from build123d import *

# Parameters (mm, degrees)
REVOLVE1_ANGLE                 = 177.5
BOSS_EXTRUDE1_REACH            = 72.435
BOSS_EXTRUDE1_END_MAJOR_RADIUS = 31.55
BOSS_EXTRUDE1_END_MINOR_RADIUS = 2.45
BOSS_EXTRUDE2_DEPTH            = 1.25
BOSS_EXTRUDE3_REACH            = 68.663
BOSS_EXTRUDE3_END_RADIUS       = 31.55
SKETCH7_R                      = 0.5
CUT_EXTRUDE1_DEPTH             = 49.523762708
BOSS_EXTRUDE4_START            = -2.45
BOSS_EXTRUDE4_DEPTH            = 4.9
BOSS_EXTRUDE5_DEPTH            = 4.9
SKETCH11_R                     = 1.05
CUT_EXTRUDE2_DEPTH             = 49.543542798
CHAMFER1_SIZE                  = 0.1
CUT_REVOLVE4_ANGLE             = 5


# Read off the part's stored shape, not the designer's step: Boss-Extrude4
with BuildPart() as part:
    # Sketch1 → Revolve1 (revolve)
    with BuildSketch(Plane(origin=(0, 0, 0), x_dir=(0, 0, -1), z_dir=(1, 0, 0))):
        with BuildLine():
            Line((-1.9, 31.55), (-2.45, 31.55))
            ThreePointArc((-2.45, 31.55), (0, 34), (2.45, 31.55))
            Line((2.45, 31.55), (1.9, 31.55))
            Line((1.9, 31.55), (1.732550899, 32.3))
            ThreePointArc((1.732550899, 32.3), (1.713964889, 32.375442776), (1.692095441, 32.45))
            ThreePointArc((1.692095441, 32.45), (0, 33.306290622), (-1.692095441, 32.45))
            ThreePointArc((-1.692095441, 32.45), (-1.713964889, 32.375442776), (-1.732550899, 32.3))
            Line((-1.732550899, 32.3), (-1.9, 31.55))
        make_face()
    revolve(axis=Axis((0, 0, -25.465534681), (0, 0, 1)), revolution_arc=REVOLVE1_ANGLE)



with BuildPart() as body_2:
    # Boss-Extrude1: up to this torus (the profile starts outside it)
    boss_extrude1_end = Plane(origin=(0, 0, 0), z_dir=(0, 0, -1)) * Torus(BOSS_EXTRUDE1_END_MAJOR_RADIUS, BOSS_EXTRUDE1_END_MINOR_RADIUS, mode=Mode.PRIVATE)
    # Sketch4 → Boss-Extrude1 (new, up to the surface)
    with BuildSketch(Plane(origin=(-11.970705016, 32.889241728, 0), x_dir=(-0.9396926207859083, -0.34202014332566943, 0), z_dir=(0.34202014332566943, -0.9396926207859083, 0)), mode=Mode.PRIVATE) as boss_extrude1_sk1:
        Polygon((3.25, 1.75), (-3.25, 1.5), (-3.25, -1.5), (3.25, -1.75), align=None)
    boss_extrude1_tool1 = extrude(boss_extrude1_sk1.sketch, amount=BOSS_EXTRUDE1_REACH, mode=Mode.PRIVATE) - boss_extrude1_end
    add(boss_extrude1_tool1.solids().sort_by_distance((-12.049013, 32.86074, 0))[0])


with BuildPart() as part_1:
    add(part.part)

    add(body_2.part)  # Boss-Extrude2 merges body 2
    # Sketch5 → Boss-Extrude2 (add, symmetric)
    with BuildSketch(Plane.XY):
        with BuildLine():
            Line((-14.896879867, 32.888378954), (-14.554859724, 31.948686333))
            Line((-14.554859724, 31.948686333), (-9.386550309, 33.829797122))
            Line((-9.386550309, 33.829797122), (-9.557560381, 34.299643432))
            Line((-9.557560381, 34.299643432), (-11.718054934, 33.513287723))
            ThreePointArc((-11.718054934, 33.513287723), (-12.14691319, 33.378696125), (-12.586125644, 33.28316224))
            Line((-12.586125644, 33.28316224), (-14.896879867, 32.888378954))
        make_face()
    extrude(amount=BOSS_EXTRUDE2_DEPTH, both=True)

    # Boss-Extrude3: up to this cylinder (the profile starts outside it)
    boss_extrude3_end = Plane(origin=(0, 0, 0), z_dir=(0, 0, -1)) * Cylinder(BOSS_EXTRUDE3_END_RADIUS, 201.426, mode=Mode.PRIVATE)
    # Sketch6 → Boss-Extrude3 (add, up to the surface)
    with BuildSketch(Plane(origin=(-17.5, 30.310889132, 0), x_dir=(0.866025403784438, 0.5000000000000012, 0), z_dir=(-0.5000000000000012, 0.866025403784438, 0)), mode=Mode.PRIVATE) as boss_extrude3_sk1:
        with BuildLine():
            Line((-0.75, -2.25), (0.75, -2.25))
            ThreePointArc((0.75, -2.25), (1.457106781, -1.957106781), (1.75, -1.25))
            Line((1.75, -1.25), (1.75, 1.25))
            ThreePointArc((1.75, 1.25), (1.457106781, 1.957106781), (0.75, 2.25))
            Line((0.75, 2.25), (-0.75, 2.25))
            ThreePointArc((-0.75, 2.25), (-1.457106781, 1.957106781), (-1.75, 1.25))
            Line((-1.75, 1.25), (-1.75, -1.25))
            ThreePointArc((-1.75, -1.25), (-1.457106781, -1.957106781), (-0.75, -2.25))
        make_face()
    boss_extrude3_tool1 = extrude(boss_extrude3_sk1.sketch, amount=-BOSS_EXTRUDE3_REACH, mode=Mode.PRIVATE) - boss_extrude3_end
    add(boss_extrude3_tool1.solids().sort_by_distance((-17.5, 30.310889, 0))[0])

    # Sketch7 → Cut-Extrude1 (cut, through all)
    with BuildSketch(Plane.XY.offset(2.25)):
        with Locations((-17, 29.444863729)):
            Circle(SKETCH7_R)
    extrude(amount=-CUT_EXTRUDE1_DEPTH, mode=Mode.SUBTRACT)

    # Boss-Extrude4 outline → Boss-Extrude4 (add)
    with BuildSketch(Plane.XY.offset(BOSS_EXTRUDE4_START)):
        with BuildLine():
            Line((-29.900129226, -17.819785976), (-27.005409062, -16.312890038))
            ThreePointArc((-27.005409062, -16.312890038), (-27.985191787, -14.568168747), (-28.852403515, -12.764846705))
            Line((-28.852403515, -12.764846705), (-31.747123679, -14.271742644))
            Line((-31.747123679, -14.271742644), (-29.900129226, -17.819785976))
        make_face()
    extrude(amount=BOSS_EXTRUDE4_DEPTH)

    # Sketch10 → Boss-Extrude5 (add)
    with BuildSketch(Plane.XY.offset(2.45)):
        with BuildLine():
            Line((-31.747123679, -14.271742644), (-29.900129226, -17.819785976))
            ThreePointArc((-29.900129226, -17.819785976), (-32.597648119, -16.969261536), (-31.747123679, -14.271742644))
        make_face()
    extrude(amount=-BOSS_EXTRUDE5_DEPTH)

    # Sketch11 → Cut-Extrude2 (cut, through all)
    with BuildSketch(Plane.XY.offset(2.45)):
        with Locations((-30.823626453, -16.04576431)):
            Circle(SKETCH11_R)
    extrude(amount=-CUT_EXTRUDE2_DEPTH, mode=Mode.SUBTRACT)

    # Chamfer1
    chamfer1_edges = [part_1.edges().sort_by_distance(p)[0] for p in [
        (-31.873626453, -16.04576431, -2.45),
        (-31.873626453, -16.04576431, 2.45),
    ]]
    chamfer(chamfer1_edges, length=CHAMFER1_SIZE)

    # Sketch12 → Cut-Revolve2 (revolve, cut)
    with BuildSketch(Plane(origin=(0, 0, 0), x_dir=(0, 0, -1), z_dir=(1, 0, 0))):
        with BuildLine():
            Line((-1.9, 31.55), (1.9, 31.55))
            Line((1.9, 31.55), (1.732550899, 32.3))
            ThreePointArc((1.732550899, 32.3), (1.713964889, 32.375442776), (1.692095441, 32.45))
            ThreePointArc((1.692095441, 32.45), (0, 33.306290622), (-1.692095441, 32.45))
            ThreePointArc((-1.692095441, 32.45), (-1.713964889, 32.375442776), (-1.732550899, 32.3))
            Line((-1.732550899, 32.3), (-1.9, 31.55))
        make_face()
    revolve(axis=Axis((0, 0, -14.066037571), (0, 0, 1)), mode=Mode.SUBTRACT)

    # Sketch13 → Cut-Revolve4 (revolve, cut)
    with BuildSketch(Plane(origin=(0, 0, 0), x_dir=(0, 0, -1), z_dir=(0.999048221581858, -0.043619387365329415, 0))):
        with BuildLine():
            Line((0, -33.306290622), (0, -34))
            ThreePointArc((0, -34), (1.732411614, -33.282411614), (2.45, -31.55))
            Line((2.45, -31.55), (1.9, -31.55))
            Line((1.9, -31.55), (1.732550899, -32.3))
            ThreePointArc((1.732550899, -32.3), (1.713964889, -32.375442776), (1.692095441, -32.45))
            ThreePointArc((1.692095441, -32.45), (0.948211555, -33.080028823), (0, -33.306290622))
        make_face()
    revolve(axis=Axis((0, 0, -14.693028928), (0, 0, -1)), revolution_arc=CUT_REVOLVE4_ANGLE, mode=Mode.SUBTRACT)


solid = part_1.part
Read the model definition and answer for the solid it produces. Units are mm, in the model's axes. A direction names the side the tool comes from. Round coordinates to 2 decimals unless told otherwise and drop trailing zeros. Write each loop counter-clockwise with the first axis right and the second up, starting at its lowest first coordinate (ties: lowest second). Pieces come first, ordered by that corner, then holes. Notation, with made-up numbers: M 81,-1.5 L 91,-1.5 A13 ccw 91,11.5 Z; hole C -26,87.5 d3. An arc over 180 degrees is marked long. Use a Markdown table: item, result.
1) Flat-ended cylindrical pins translate along their axes: pin 1 (2 mm diameter, centred on x = -29, z = -0.5, fed in from -Y); pin 2 (1.9 mm diameter, centred on x = -11.5, y = 33, fed in from -Z); pin 3 (3 mm diameter, centred on x = -17.5, y = 28.5, fed in from +Z). Find the tip coordinate at first contact, or state that the pin passes through.
Answers follow:
| item | result |
|---|---|
| pin 1 | stops at y = -19.23 |
| pin 2 | stops at z = -1.64 |
| pin 3 | stops at z = 2.42 |
2) The part is cut by section A-A (y = 0). Write down the section's boundary in (x, z).
Answers follow:
| item | result |
|---|---|
| outline | M -32.45,-1.69 A2.1 cw -32.45,1.69 A1.78 cw -32.3,1.73 L -31.55,1.9 L -31.55,2.45 A2.45 ccw -31.55,-2.45 L -31.55,-1.9 L -32.3,-1.73 A1.78 cw Z |
3) Straight lines are drawn through the part: line 1 along Y through (x, z) = (-17, 0.45); line 2 along Y through (x, z) = (-14.5, -0.3); line 3 along Y through (x, z) = (-29, 1.05). For each, find the intervals that lie inside material, in ascending order. Write a range as [from, to].
Answers follow:
| item | result |
|---|---|
| line 1 | y = [-29.4, -28.58], [28.58, 28.94], [29.94, 30.6] |
| line 2 | y = [-30.73, -29.96], [29.96, 32.96] |
| line 3 | y = [-17.35, -15.8], [15.8, 17.29] |
4) For a pull along Y with two mould halves and no side action, classify faces 4 (the flat face through (-1.446, -33.112, 1.31)), 5 (the flat face through (-8.7, 33.4, 0)), 6 (the flat face through (-30, -15, -2.45)), 7 (the cylindrical face through (-31.873, -16, 0.033)) as pulls with the +Y half, pulls with the -Y half, needs draft (parallel to the pull), parting line crosses it, or undercut.
Answers follow:
| item | result |
|---|---|
| face 4 | pulls with the -Y half |
| face 5 | pulls with the +Y half |
| face 6 | needs draft |
| face 7 | undercut |
5) A tool of negligible diameter and unlimited length cuts with its end or side. For faces 1 (the flat face through (-29.44, -17.58, -0.03)), 2 (the cylindrical face through (-15.77, 30.212, 1.965)), 3 (the flat face through (-16.6, 28.8, -2.25)), from which of +Z, -Z, +X, -X, +Y, -Y can it reach the whole face along a straight path? Write none if from no direction.
Answers follow:
| item | result |
|---|---|
| face 1 | -Y |
| face 2 | +Z, +Y |
| face 3 | -Z, -X, +Y |
